Can you work these out from the model? Positions are in its coordinate system, mm. A direction names the side the tool comes from. Coordinates: 2 decimals unless noted, no trailing zeros. Write each loop counter-clockwise with the first axis right and the second up, starting at its lowest first coordinate (ties: lowest second). Pieces come first, ordered by that corner, then holes. Notation, with made-up numbers: (-24, -23) - (13, -23) arc R13 cw to (13, -17) - close; hole circle Ø10 at (53.25, -6). An arc over 180 degrees is marked (long way). One line per question, with ' | ' between items. Start each with the question number.
from build123d import *

# Parameters (mm, degrees)
BOSS_EXTRUDE1_DEPTH = 5
FILLET1_R           = 4
SKETCH2_R           = 3
CUT_EXTRUDE1_DEPTH  = 41.614036982
SKETCH3_R           = 28.5
BOSS_EXTRUDE2_DEPTH = 45
SKETCH4_R           = 19
BOSS_EXTRUDE3_DEPTH = 1.5
SKETCH5_R           = 4.5
CUT_EXTRUDE2_DEPTH  = 3
SKETCH6_R           = 3
CUT_EXTRUDE3_DEPTH  = 64.06147794


with BuildPart() as part:
    # Sketch1 → Boss-Extrude1 (new body)
    with BuildSketch(Plane(origin=(0, 0, 0), x_dir=(1, 0, 0), z_dir=(0, 1, 0))):
        Polygon((-28.5, 0), (-28.5, 28.5), (28.5, 28.5), (28.5, -28.5), (-28.5, -28.5), align=None)
    extrude(amount=BOSS_EXTRUDE1_DEPTH)

    # Fillet1
    fillet1_edges = [part.edges().sort_by_distance(p)[0] for p in [
        (-28.5, 2.5, -28.5),
        (28.5, 2.5, -28.5),
        (28.5, 2.5, 28.5),
        (-28.5, 2.5, 28.5),
    ]]
    fillet(fillet1_edges, radius=FILLET1_R)

    # Sketch2 → Cut-Extrude1 (cut, through all)
    with BuildSketch(Plane(origin=(0, 5, 0), x_dir=(1, 0, 0), z_dir=(0, 1, 0))):
        with Locations(Location((-23.5, 23.5, 0), (0, 0, 270))):
            Circle(SKETCH2_R)
        with Locations(Location((23.5, 23.5, 0), (0, 0, 270))):
            Circle(SKETCH2_R)
        with Locations(Location((23.5, -23.5, 0), (0, 0, 270))):
            Circle(SKETCH2_R)
        with Locations(Location((-23.5, -23.5, 0), (0, 0, 270))):
            Circle(SKETCH2_R)
    extrude(amount=-CUT_EXTRUDE1_DEPTH, mode=Mode.SUBTRACT)

    # Sketch3 → Boss-Extrude2 (add)
    with BuildSketch(Plane.XZ):
        with Locations(Location((0, 0, 0), (0, 0, 270))):
            Circle(SKETCH3_R)
    extrude(amount=BOSS_EXTRUDE2_DEPTH)

    # Sketch4 → Boss-Extrude3 (add)
    with BuildSketch(Plane(origin=(0, 5, 0), x_dir=(1, 0, 0), z_dir=(0, 1, 0))):
        with Locations(Location((0, 0, 0), (0, 0, 90))):
            Circle(SKETCH4_R)
    extrude(amount=BOSS_EXTRUDE3_DEPTH)

    # Sketch5 → Cut-Extrude2 (cut)
    with BuildSketch(Plane(origin=(0, 6.5, 0), x_dir=(1, 0, 0), z_dir=(0, 1, 0))):
        with Locations(Location((0, 0, 0), (0, 0, 270))):
            Circle(SKETCH5_R)
    extrude(amount=-CUT_EXTRUDE2_DEPTH, mode=Mode.SUBTRACT)

    # Sketch6 → Cut-Extrude3 (cut, through all)
    with BuildSketch(Plane(origin=(0, 3.5, 0), x_dir=(1, 0, 0), z_dir=(0, 1, 0))):
        with Locations(Location((0, 0, 0), (0, 0, 270))):
            Circle(SKETCH6_R)
    extrude(amount=-CUT_EXTRUDE3_DEPTH, mode=Mode.SUBTRACT)


solid = part.part
(1) If we section it at D-D on y = -34.5: List the corners of the cut face in (x, z) for me.
(2) Which directions (+Z, -Z, +X, -X, +Y, -Y) give clear straight access to the entire face, cutting with the end or side of a thin tool? Please do faces 1 (the face through (11.56, 5.74, 15.08)), 2 (the face through (-21, 0, -21)), 3 (the face through (20.6, 0, -21.7)), 4 (the face through (-27.359, 2.535, -27.297)), 5 (the face through (21.7, 0, 20.5)).
(3) I'm going to push flat-ended pins straight in: pin 1 (5 mm diameter, centred on x = -23.5, z = 23.5, fed in from -Y); pin 2 (1.5 mm diameter, centred on x = 3.5, y = -10, fed in from +Z); pin 3 (5 mm diameter, centred on x = -16.5, y = -30.5, fed in from -Z); pin 4 (5 mm diameter, centred on x = -13, y = -18.5, fed in from +Z). Where does each tip first touch, or does it pass through?
(4) If we section it at B-B on z = -23.5: List the corners of the cut face in (x, y) for me, plus the area to 3 significant figures.
(5) If we mould it in two halves opening along Z, with no side actions, what happens to faces 6 (the face through (0.9, -20.41, 2.86)), 7 (the face through (-20.5, 0, 21.6)), 8 (the face through (-27.82, -22.18, 6.18))? For each: +Z half, -Z half, draft (parallel to the pull), parting line (faces both ways), or undercut.
(6) If we section it at A-A on x = -23.5: List the corners of the cut face in (y, z) for me.
(7) If I drill on probe 1 along X at (y, z) = (1, 23); probe 2 along X at (y, z) = (-23, 0); probe 3 along Y at (x, z) = (24.5, -6), over which ranges is the centre line in solid material (lowest first)?
Values:
1) outline: circle Ø57 at (0, 0); hole circle Ø6 at (0, 0)
2) face 1: +Y | face 2: -Z, -X, -Y | face 3: -Z, +X, -Y | face 4: -Z, -X, +Y, -Y | face 5: +Z, +X, -Y
3) pin 1: through | pin 2: z = 28.37 | pin 3: z = -24.82 | pin 4: z = 26.5
4) outline: (-28.5, 0) - (-26.5, 0) - (-26.5, 5) - (-28.5, 5) - close; (-20.5, 0) - (-16.12, 0) - (-16.12, -45) - (16.12, -45) - (16.12, 0) - (20.5, 0) - (20.5, 5) - (-20.5, 5) - close; (26.5, 0) - (28.5, 0) - (28.5, 5) - (26.5, 5) - close | area: 1,680 mm2
5) face 6: undercut | face 7: draft | face 8: parting line
6) outline: (-45, -16.12) - (0, -16.12) - (0, -20.5) - (5, -20.5) - (5, 20.5) - (0, 20.5) - (0, 16.12) - (-45, 16.12) - close; (0, -28.5) - (5, -28.5) - (5, -26.5) - (0, -26.5) - close; (0, 26.5) - (5, 26.5) - (5, 28.5) - (0, 28.5) - close
7) probe 1: -28.5 to -26.46, -20.54 to 20.54, 26.46 to 28.5 | probe 2: -28.5 to -3, 3 to 28.5 | probe 3: -45 to 5
